Build history of the part. All positions in model axes, mm. A direction names the side the tool comes from. Round coordinates to 2 decimals unless told otherwise and drop trailing zeros. Order: outer loops, then holes, each group sorted by start corner. A loop starts at its lowest first (then second) coordinate and runs counter-clockwise, first axis right, second up. Notation, with made-up numbers: (-5, 15.25) -> (7, 15.25) arc R29 cw to (7, 38.25) -> close; hole circle Ø3 at (-15.5, -20.75). An arc over 180 degrees is marked (long way). Use a Markdown table: item, result. Add a question column.
Item 1: Slice it at B-B, the plane x = 16.5. Give the cut face in (y, z), plus the area to 3 significant figures.
Item 2: Slice it at C-C, the plane y = -11. Give the cut face in (x, z), plus the area to 3 significant figures.
Item 3: Pin check, flat tips, straight feed: pin 1 (12 mm diameter, centred on x = 27.5, z = 43, fed in from -Y); pin 2 (9 mm diameter, centred on x = 0, z = 31, fed in from -Y); pin 3 (8 mm diameter, centred on x = -22, z = 22, fed in from +Y). Stop position of each tip, or through.
Item 4: Probe L1, parallel to Y at x = -10.5, z = 52; L2, parallel to Y at x = 0, z = 0.7; L3, parallel to Y at x = 38.5, z = 14.5. List the from-to ranges inside material, lowest first.
Item 5: Slice it at A-A, the plane y = 36. Give the cut face in (x, z), plus the area to 3 significant figures.
Item 6: Slice it at D-D, the plane z = 48.5. State how many separate pieces and enclosed holes the cut face has, plus the area to 3 significant figures.
Item 7: Two-plate mould, pull along Y, no slides. Class faces 4 (the face through (22.967, -38.698, 29.58)), 5 (the face through (0.4, -4.5, 60)): released by +Y, released by -Y, zero draft, split by the parting line, or undercut.
Item 8: 3-axis set-ups, long thin cutter, end or side, ignore diameter. For faces 1 (the face through (-7.281, -44.407, 29.58)), 2 (the face through (-0.67, -7.97, 32.62)), 3 (the face through (4.867, -2.018, 7.769)): which of +Z, -Z, +X, -X, +Y, -Y reach the whole face in a straight line?
from build123d import *

# Parameters (mm, degrees)
CYLINDER021_R          = 7
CYLINDER021_DEPTH      = 2
TUBE017_R              = 60
TUBE017_R_2            = 46
TUBE017_DEPTH          = 60
BOX028_W               = 8.4
BOX028_H               = 8.4
BOX028_DEPTH           = 60
CYLINDER020_R          = 8
CYLINDER020_DEPTH      = 60
TUBE016_R              = 46
TUBE016_R_2            = 45
TUBE016_DEPTH          = 60
BOX029_W               = 50
BOX029_H               = 1.5
BOX029_DEPTH           = 60
BOX029_PLACEMENT_ANGLE = 40
BOX030_W               = 50
BOX030_H               = 1.5
BOX030_DEPTH           = 60
BOX030_PLACEMENT_ANGLE = 80
BOX031_W               = 50
BOX031_H               = 1.5
BOX031_DEPTH           = 60
BOX031_PLACEMENT_ANGLE = 120
BOX032_W               = 50
BOX032_H               = 1.5
BOX032_DEPTH           = 60
BOX032_PLACEMENT_ANGLE = 160
BOX033_W               = 50
BOX033_H               = 1.5
BOX033_DEPTH           = 60
BOX033_PLACEMENT_ANGLE = 200
BOX034_W               = 50
BOX034_H               = 1.5
BOX034_DEPTH           = 60
BOX034_PLACEMENT_ANGLE = 40
BOX035_W               = 50
BOX035_H               = 1.5
BOX035_DEPTH           = 60
BOX035_PLACEMENT_ANGLE = 280
BOX036_W               = 50
BOX036_H               = 1.5
BOX036_DEPTH           = 60
BOX036_PLACEMENT_ANGLE = 240
BOX037_W               = 50
BOX037_H               = 1.5
BOX037_DEPTH           = 60
BOX037_PLACEMENT_ANGLE = 200
BOX026_W               = 50
BOX026_H               = 1.5
BOX026_DEPTH           = 60


with BuildPart() as cone005:
    # Cone005 → Cone005 (revolve)
    with BuildSketch(Plane(origin=(0, 0, 2), x_dir=(1, 0, 0), z_dir=(0, -1, 0))):
        Polygon((0, 0), (7, 0), (4, 10), (0, 10), align=None)
    revolve(axis=Axis((0, 0, 2), (0, 0, 1)))


with BuildPart() as cylinder021:
    # Cylinder021 → Cylinder021 (new body)
    with BuildSketch(Plane.XY):
        Circle(CYLINDER021_R)
    extrude(amount=CYLINDER021_DEPTH)


with BuildPart() as tube017:
    # Tube017 → Tube017 (new body)
    with BuildSketch(Plane.XY):
        Circle(TUBE017_R)
        Circle(TUBE017_R_2, mode=Mode.SUBTRACT)
    extrude(amount=TUBE017_DEPTH)


with BuildPart() as fusion009008:
    # Box028 → Box028 (new body)
    with BuildSketch(Plane(origin=(-4.2, -4.2, 0), x_dir=(1, 0, 0), z_dir=(0, 0, 1))):
        with Locations((4.2, 4.2)):
            Rectangle(BOX028_W, BOX028_H)
    extrude(amount=BOX028_DEPTH)

    # Fusion009008: union Cone005, Cylinder021, Tube017
    add(cone005.part)
    add(cylinder021.part)
    add(tube017.part)


with BuildPart() as cylinder020:
    # Cylinder020 → Cylinder020 (new body)
    with BuildSketch(Plane.XY):
        Circle(CYLINDER020_R)
    extrude(amount=CYLINDER020_DEPTH)


with BuildPart() as tube016:
    # Tube016 → Tube016 (new body)
    with BuildSketch(Plane.XY):
        Circle(TUBE016_R)
        Circle(TUBE016_R_2, mode=Mode.SUBTRACT)
    extrude(amount=TUBE016_DEPTH)


with BuildPart() as cone006:
    # Cone006 → Cone006 (revolve)
    with BuildSketch(Plane.XZ):
        Polygon((0, 0), (9, 0), (4, 30), (0, 30), align=None)
    revolve(axis=Axis((0, 0, 0), (0, 0, 1)))


with BuildPart() as cube029:
    # Box029 → Box029 (new body)
    with BuildSketch(Plane.XY):
        with Locations((25, 0.75)):
            Rectangle(BOX029_W, BOX029_H)
    extrude(amount=BOX029_DEPTH)


with BuildPart() as cube029_1:
    # Box029 placement: moved
    add(cube029.part.rotate(Axis((0, 0, 0), (0, 0, 1)), BOX029_PLACEMENT_ANGLE))


with BuildPart() as cube030:
    # Box030 → Box030 (new body)
    with BuildSketch(Plane.XY):
        with Locations((25, 0.75)):
            Rectangle(BOX030_W, BOX030_H)
    extrude(amount=BOX030_DEPTH)


with BuildPart() as cube030_1:
    # Box030 placement: moved
    add(cube030.part.rotate(Axis((0, 0, 0), (0, 0, 1)), BOX030_PLACEMENT_ANGLE))


with BuildPart() as cube031:
    # Box031 → Box031 (new body)
    with BuildSketch(Plane.XY):
        with Locations((25, 0.75)):
            Rectangle(BOX031_W, BOX031_H)
    extrude(amount=BOX031_DEPTH)


with BuildPart() as cube031_1:
    # Box031 placement: moved
    add(cube031.part.rotate(Axis((0, 0, 0), (0, 0, 1)), BOX031_PLACEMENT_ANGLE))


with BuildPart() as cube032:
    # Box032 → Box032 (new body)
    with BuildSketch(Plane.XY):
        with Locations((25, 0.75)):
            Rectangle(BOX032_W, BOX032_H)
    extrude(amount=BOX032_DEPTH)


with BuildPart() as cube032_1:
    # Box032 placement: moved
    add(cube032.part.rotate(Axis((0, 0, 0), (0, 0, 1)), BOX032_PLACEMENT_ANGLE))


with BuildPart() as cube033:
    # Box033 → Box033 (new body)
    with BuildSketch(Plane.XY):
        with Locations((25, 0.75)):
            Rectangle(BOX033_W, BOX033_H)
    extrude(amount=BOX033_DEPTH)


with BuildPart() as cube033_1:
    # Box033 placement: moved
    add(cube033.part.rotate(Axis((0, 0, 0), (0, 0, 1)), BOX033_PLACEMENT_ANGLE))


with BuildPart() as cube034:
    # Box034 → Box034 (new body)
    with BuildSketch(Plane.XY):
        with Locations((25, 0.75)):
            Rectangle(BOX034_W, BOX034_H)
    extrude(amount=BOX034_DEPTH)


with BuildPart() as cube034_1:
    # Box034 placement: moved
    add(cube034.part.rotate(Axis((0, 0, 0), (0, 0, -1)), BOX034_PLACEMENT_ANGLE))


with BuildPart() as cube035:
    # Box035 → Box035 (new body)
    with BuildSketch(Plane.XY):
        with Locations((25, 0.75)):
            Rectangle(BOX035_W, BOX035_H)
    extrude(amount=BOX035_DEPTH)


with BuildPart() as cube035_1:
    # Box035 placement: moved
    add(cube035.part.rotate(Axis((0, 0, 0), (0, 0, 1)), BOX035_PLACEMENT_ANGLE))


with BuildPart() as cube036:
    # Box036 → Box036 (new body)
    with BuildSketch(Plane.XY):
        with Locations((25, 0.75)):
            Rectangle(BOX036_W, BOX036_H)
    extrude(amount=BOX036_DEPTH)


with BuildPart() as cube036_1:
    # Box036 placement: moved
    add(cube036.part.rotate(Axis((0, 0, 0), (0, 0, 1)), BOX036_PLACEMENT_ANGLE))


with BuildPart() as cube037:
    # Box037 → Box037 (new body)
    with BuildSketch(Plane.XY):
        with Locations((25, 0.75)):
            Rectangle(BOX037_W, BOX037_H)
    extrude(amount=BOX037_DEPTH)


with BuildPart() as cube037_1:
    # Box037 placement: moved
    add(cube037.part.rotate(Axis((0, 0, 0), (0, 0, 1)), BOX037_PLACEMENT_ANGLE))


with BuildPart() as obj1:
    # Box026 → Box026 (new body)
    with BuildSketch(Plane.XY):
        with Locations((25, 0.75)):
            Rectangle(BOX026_W, BOX026_H)
    extrude(amount=BOX026_DEPTH)

    # Fusion009009: union Cylinder020, Tube016, Cone006, Cube029, Cube030, Cube031, Cube032, Cube033, Cube034, Cube035, Cube036, Cube037
    add(cylinder020.part)
    add(tube016.part)
    add(cone006.part)
    add(cube029_1.part)
    add(cube030_1.part)
    add(cube031_1.part)
    add(cube032_1.part)
    add(cube033_1.part)
    add(cube034_1.part)
    add(cube035_1.part)
    add(cube036_1.part)
    add(cube037_1.part)

    # Cut009008: cut Fusion009008
    add(fusion009008.part, mode=Mode.SUBTRACT)


solid = obj1.part
Check sheet entries:
| question | item | result |
|---|---|---|
| 1 | outline | (-42.94, 0) -> (-41.87, 0) -> (-41.87, 60) -> (-42.94, 60) -> close; (-13.85, 0) -> (-11.89, 0) -> (-11.89, 60) -> (-13.85, 60) -> close; (0, 0) -> (1.5, 0) -> (1.5, 60) -> (0, 60) -> close; (13.85, 0) -> (15.8, 0) -> (15.8, 60) -> (13.85, 60) -> close; (41.87, 0) -> (42.94, 0) -> (42.94, 60) -> (41.87, 60) -> close |
| 1 | area | 454 mm2 |
| 2 | outline | (-44.67, 0) -> (-43.63, 0) -> (-43.63, 60) -> (-44.67, 60) -> close; (-30.22, 0) -> (-25.84, 0) -> (-25.84, 60) -> (-30.22, 60) -> close; (-6.35, 0) -> (-4.62, 0) -> (-4.62, 60) -> (-6.35, 60) -> close; (1.94, 0) -> (3.46, 0) -> (3.46, 60) -> (1.94, 60) -> close; (13.11, 0) -> (15.44, 0) -> (15.44, 60) -> (13.11, 60) -> close; (43.63, 0) -> (44.67, 0) -> (44.67, 60) -> (43.63, 60) -> close |
| 2 | area | 722 mm2 |
| 3 | pin 1 | y = -40.67 |
| 3 | pin 2 | y = -46 |
| 3 | pin 3 | y = 42.33 |
| 4 | L1 | -44.79 to -43.76, -21.19 to -18.19, -5.42 to -3.82, 2.23 to 3.82, 15.19 to 18.19, 43.76 to 44.79 |
| 4 | L2 | -46 to -45, -8.88 to -7, 7 to 8.88, 45 to 46 |
| 4 | L3 | -25.17 to -23.3, 0 to 1.5, 23.3 to 25.17 |
| 5 | outline | (-28.64, 0) -> (-27, 0) -> (-27, 60) -> (-28.64, 60) -> close; (-22.52, 0) -> (-20.78, 0) -> (-20.78, 60) -> (-22.52, 60) -> close; (4.82, 0) -> (6.35, 0) -> (6.35, 60) -> (4.82, 60) -> close; (27, 0) -> (28.64, 0) -> (28.64, 60) -> (27, 60) -> close |
| 5 | area | 392 mm2 |
| 6 | separate pieces | 1 |
| 6 | enclosed holes | 10 |
| 6 | area | 916 mm2 |
| 7 | face 4 | undercut |
| 7 | face 5 | zero draft |
| 8 | face 1 | +Z, -Z |
| 8 | face 2 | +Z |
| 8 | face 3 | -Z |
